from build123d import *
from OCP.BRepFilletAPI import BRepFilletAPI_MakeChamfer

# Parameters (mm, degrees)
BASE_FLANGE1_DEPTH             = 70
SKETCH7_W                      = 25
SKETCH7_H                      = 20
CUT_EXTRUDE1_DEPTH             = 90.017176187
MIRROR10_COPY_1_SKETCH_W       = 25
MIRROR10_COPY_1_SKETCH_H       = 20
MIRROR10_COPY_1_DEPTH          = 90.017176187
FILLET3_R                      = 10
FILLET4_R                      = 2
TAP_DRILL_FOR_4_40_TAP1_D      = 2.2606
SKETCH11_R                     = 5
CUT_EXTRUDE2_DEPTH             = 10
CUT_EXTRUDE3_DEPTH             = 10
CIRPATTERN1_COUNT              = 6
F_5_16_0_3125_DIAMETER_HOLE1_D = 7.9375
TAP_DRILL_FOR_M3X0_5_TAP1_D    = 2.5
CIRPATTERN2_COUNT              = 4
CHAMFER2_SIZE                  = 17
CHAMFER2_SIZE2                 = 9.814954576
FILLET5_R                      = 3
CHAMFER3_SIZE                  = 17
CHAMFER3_SIZE2                 = 9.814954576
FILLET6_R                      = 3


# Sheet-metal steps are written as plain solids
with BuildPart() as part:
    # Sketch2 → Base-Flange1 (new body)
    with BuildSketch(Plane.XY):
        with BuildLine():
            Line((-44.5, 30), (-44.5, 0.7366))
            ThreePointArc((-44.5, 0.7366), (-44.284254855, 0.215745145), (-43.7634, 0))
            Line((-43.7634, 0), (43.7634, 0))
            ThreePointArc((43.7634, 0), (44.284254855, 0.215745145), (44.5, 0.7366))
            Line((44.5, 0.7366), (44.5, 30))
            Line((44.5, 30), (46.0875, 30))
            Line((46.0875, 30), (46.0875, 0.7366))
            ThreePointArc((46.0875, 0.7366), (45.40678687, -0.90678687), (43.7634, -1.5875))
            Line((43.7634, -1.5875), (-43.7634, -1.5875))
            ThreePointArc((-43.7634, -1.5875), (-45.40678687, -0.90678687), (-46.0875, 0.7366))
            Line((-46.0875, 0.7366), (-46.0875, 30))
            Line((-46.0875, 30), (-44.5, 30))
        make_face()
    extrude(amount=BASE_FLANGE1_DEPTH)

    # Sketch7 → Cut-Extrude1 (cut, symmetric)
    with BuildSketch(Plane(origin=(0, 0, 0), x_dir=(1, 0, 0), z_dir=(0, 1, 0))):
        with Locations((-33.5875, -60)):
            Rectangle(SKETCH7_W, SKETCH7_H)
    cut_extrude1 = extrude(amount=CUT_EXTRUDE1_DEPTH, both=True, mode=Mode.SUBTRACT)

    # Mirror9: Cut-Extrude1 across plane
    add(cut_extrude1.mirror(Plane.ZY), mode=Mode.SUBTRACT)

    # Mirror10: Cut-Extrude1 across plane
    add(cut_extrude1.mirror(Plane(origin=(0, 0, 35), x_dir=(1, 0, 0), z_dir=(0, 0, -1))), mode=Mode.SUBTRACT)

    # Mirror10 copy 1 sketch → Mirror10 copy 1 (cut, symmetric)
    with BuildSketch(Plane(origin=(0, 0, 70), x_dir=(-1, 0, 0), z_dir=(0, 1, 0))):
        with Locations((-33.5875, -60)):
            Rectangle(MIRROR10_COPY_1_SKETCH_W, MIRROR10_COPY_1_SKETCH_H)
    extrude(amount=MIRROR10_COPY_1_DEPTH, both=True, mode=Mode.SUBTRACT)

    # Fillet3
    fillet3_edges = [part.edges().sort_by_distance(p)[0] for p in [
        (21.0875, -0.79375, 0),
        (-21.0875, -0.79375, 0),
        (-21.0875, -0.79375, 70),
        (21.0875, -0.79375, 70),
    ]]
    fillet(fillet3_edges, radius=FILLET3_R)

    # Fillet4
    fillet4_edges = [part.edges().sort_by_distance(p)[0] for p in [
        (21.0875, -0.79375, 20),
        (-21.0875, -0.79375, 20),
        (-21.0875, -0.79375, 50),
        (21.0875, -0.79375, 50),
    ]]
    fillet(fillet4_edges, radius=FILLET4_R)

    # Tap Drill for #4-40 Tap1 (through all)
    with Locations(Plane(origin=(0, 0, 0), x_dir=(1, 0, 0), z_dir=(0, 1, 0))):
        with Locations((0.5, -10), (0.5, -60), (-34.5, -35), (35.5, -35), (-14.74, -60), (15.74, -60), (-14.74, -10), (15.74, -10)):
            Hole(TAP_DRILL_FOR_4_40_TAP1_D / 2)

    # Sketch11 → Cut-Extrude2 (cut)
    with BuildSketch(Plane(origin=(0, 0, 0), x_dir=(1, 0, 0), z_dir=(0, 1, 0))):
        with Locations(Location((-0.5, -35, 0), (0, 0, 270))):
            Circle(SKETCH11_R)
    extrude(amount=-CUT_EXTRUDE2_DEPTH, mode=Mode.SUBTRACT)

    # Sketch12 → Cut-Extrude3 (cut)
    with BuildSketch(Plane(origin=(0, 0, 0), x_dir=(1, 0, 0), z_dir=(0, 1, 0))):
        with BuildLine():
            Line((9.5, -33), (19.5, -33))
            ThreePointArc((19.5, -33), (21.5, -35), (19.5, -37))
            Line((19.5, -37), (9.5, -37))
            ThreePointArc((9.5, -37), (7.5, -35), (9.5, -33))
        make_face()
    cut_extrude3 = extrude(amount=-CUT_EXTRUDE3_DEPTH, mode=Mode.SUBTRACT)

    # CirPattern1: Cut-Extrude3 ×6 about axis
    cirpattern1_axis = Axis((-0.5, 0, 35), (0, 1, 0))
    for i in range(1, CIRPATTERN1_COUNT):
        add(cut_extrude3.rotate(cirpattern1_axis, i * 360 / CIRPATTERN1_COUNT), mode=Mode.SUBTRACT)

    # 5/16 (0.3125) Diameter Hole1 (through all)
    with Locations(Plane(origin=(46.0875, 0, 0), x_dir=(0, 0, -1), z_dir=(1, 0, 0))):
        with Locations((-35, 20)):
            Hole(F_5_16_0_3125_DIAMETER_HOLE1_D / 2)

    # Tap Drill for M3x0.5 Tap1 (through all)
    with Locations(Plane(origin=(46.0875, 0, 0), x_dir=(0, 0, -1), z_dir=(1, 0, 0))):
        with Locations((-35, 13)):
            tap_drill_for_m3x0_5_tap1 = Hole(TAP_DRILL_FOR_M3X0_5_TAP1_D / 2)

    # CirPattern2: Tap Drill for M3x0.5 Tap1 ×4 about axis
    cirpattern2_axis = Axis((0, 20, 35), (1, 0, 0))
    for i in range(1, CIRPATTERN2_COUNT):
        add(tap_drill_for_m3x0_5_tap1.rotate(cirpattern2_axis, i * 360 / CIRPATTERN2_COUNT), mode=Mode.SUBTRACT)

    # Chamfer2: one chamfer whose edges measure the first distance from different faces: ONE call of the kernel's chamfer builder (chamfer() names one face for all edges)
    chamfer2_edges_1 = [part.edges().sort_by_distance(p)[0] for p in [
        (45.29375, 30, 20),
    ]]
    chamfer2_side_1 = [part.faces().sort_by_distance(p)[0] for p in [
        (33.42545, -0.390739063, 20),
    ]]
    chamfer2_edges_2 = [part.edges().sort_by_distance(p)[0] for p in [
        (45.29375, 30, 50),
    ]]
    chamfer2_side_2 = [part.faces().sort_by_distance(p)[0] for p in [
        (33.42545, -0.390739063, 50),
    ]]
    chamfer2 = BRepFilletAPI_MakeChamfer(part.part.solid().wrapped)
    for e in chamfer2_edges_1:
        chamfer2.Add(CHAMFER2_SIZE, CHAMFER2_SIZE2, e.wrapped, chamfer2_side_1[0].wrapped)  # the first distance lies on this face
    for e in chamfer2_edges_2:
        chamfer2.Add(CHAMFER2_SIZE, CHAMFER2_SIZE2, e.wrapped, chamfer2_side_2[0].wrapped)  # the first distance lies on this face
    add(Compound.cast(chamfer2.Shape()), mode=Mode.REPLACE)

    # Fillet5
    fillet5_edges = [part.edges().sort_by_distance(p)[0] for p in [
        (45.29375, 13, 20),
        (45.29375, 30, 40.185045424),
        (45.29375, 30, 29.814954576),
        (45.29375, 13, 50),
    ]]
    fillet(fillet5_edges, radius=FILLET5_R)

    # Chamfer3: one chamfer whose edges measure the first distance from different faces: ONE call of the kernel's chamfer builder (chamfer() names one face for all edges)
    chamfer3_edges_1 = [part.edges().sort_by_distance(p)[0] for p in [
        (-45.29375, 30, 20),
    ]]
    chamfer3_side_1 = [part.faces().sort_by_distance(p)[0] for p in [
        (-33.42545, -0.390739063, 20),
    ]]
    chamfer3_edges_2 = [part.edges().sort_by_distance(p)[0] for p in [
        (-45.29375, 30, 50),
    ]]
    chamfer3_side_2 = [part.faces().sort_by_distance(p)[0] for p in [
        (-33.42545, -0.390739063, 50),
    ]]
    chamfer3 = BRepFilletAPI_MakeChamfer(part.part.solid().wrapped)
    for e in chamfer3_edges_1:
        chamfer3.Add(CHAMFER3_SIZE, CHAMFER3_SIZE2, e.wrapped, chamfer3_side_1[0].wrapped)  # the first distance lies on this face
    for e in chamfer3_edges_2:
        chamfer3.Add(CHAMFER3_SIZE, CHAMFER3_SIZE2, e.wrapped, chamfer3_side_2[0].wrapped)  # the first distance lies on this face
    add(Compound.cast(chamfer3.Shape()), mode=Mode.REPLACE)

    # Fillet6
    fillet6_edges = [part.edges().sort_by_distance(p)[0] for p in [
        (-45.29375, 13, 50),
        (-45.29375, 30, 29.814954576),
        (-45.29375, 30, 40.185045424),
        (-45.29375, 13, 20),
    ]]
    fillet(fillet6_edges, radius=FILLET6_R)


solid = part.part
Read the model definition and answer for the solid it produces. Units are mm, in the model's axes. A direction names the side the tool comes from. Give positions to 0.01 mm unless a question says otherwise; leave off trailing zeros. Loops run counter-clockwise (first coordinate to the right, second up) from the corner with the lowest first, then second, coordinate; pieces in that order, holes last. Notation, with made-up numbers: (72, -12.5) -> (125, -12.5) arc R13 cw to (125, -8.5) -> close; hole circle Ø4 at (86.25, 10.5). An arc over 180 degrees is marked (long way). Use a Markdown table: item, result.
Q1. Determine the mould class of faces 1 (the face through (-8.5, -0.8, 35)), 2 (the face through (46.088, 15.6, 34.8)), 3 (the face through (-38.9, -0.3, 20)) for opening direction X: pulls with the +X half, pulls with the -X half, needs draft (parallel to the pull), parting line crosses it, or undercut.
Solved:
| item | result |
|---|---|
| face 1 | undercut |
| face 2 | pulls with the +X half |
| face 3 | needs draft |
Q2. A tool of negligible diameter and unlimited length cuts with its end or side. For faces 4 (the face through (45.28, 14.24, 34.84)), 5 (the face through (-9.697, -0.783, 23.07)), 6 (the face through (-44.5, 15.6, 34.8)), from which of +Z, -Z, +X, -X, +Y, -Y can it reach the whole face along a straight path? Write none if from no direction.
Solved:
| item | result |
|---|---|
| face 4 | +X, -X |
| face 5 | +Y, -Y |
| face 6 | +Z, -Z, +Y |
Q3. Section B-B, the plane x = 15.74 is taken. Determine the outline of the cut face in (y, z).
Solved:
| item | result |
|---|---|
| outline | (-1.59, 1.15) -> (0, 1.15) -> (0, 8.87) -> (-1.59, 8.87) -> close; (-1.59, 11.13) -> (0, 11.13) -> (0, 33) -> (-1.59, 33) -> close; (-1.59, 37) -> (0, 37) -> (0, 58.87) -> (-1.59, 58.87) -> close; (-1.59, 61.13) -> (0, 61.13) -> (0, 68.85) -> (-1.59, 68.85) -> close |
Q4. Each of these flat-tipped pins is pushed along its axis until it touches: pin 1 (2 mm diameter, centred on x = -34.5, z = 35, fed in from -Y); pin 2 (2.5 mm diameter, centred on x = 0.5, z = 60, fed in from +Y); pin 3 (4 mm diameter, centred on y = 27, z = 35, fed in from +X); pin 4 (1.7 mm diameter, centred on y = -0.5, z = 55, fed in from -X). Where does it stop, or does it pass through?
Solved:
| item | result |
|---|---|
| pin 1 | passes through |
| pin 2 | stops at y = 0 |
| pin 3 | stops at x = 46.09 |
| pin 4 | stops at x = -21.09 |
Q5. Section A-A, the plane x = 35.5 is taken. Determine the outline of the cut face in (y, z).
Solved:
| item | result |
|---|---|
| outline | (-1.59, 20) -> (0, 20) -> (0, 33.87) -> (-1.59, 33.87) -> close; (-1.59, 36.13) -> (0, 36.13) -> (0, 50) -> (-1.59, 50) -> close |
Q6. Section C-C, the plane y = 20 is taken. Count the separate pieces of the cut face and the enclosed holes in it, then the cut area to 3 significant figures.
Solved:
| item | result |
|---|---|
| separate pieces | 8 |
| enclosed holes | 0 |
| area | 28.5 mm^2 |
Q7. Section D-D, the plane z = 24 is taken. Determine the outline of the cut face in (x, y), then the cut area to 3 significant figures.
Solved:
| item | result |
|---|---|
| outline | (-46.09, 0.74) arc R2.32 ccw to (-43.76, -1.59) -> (-9.16, -1.59) -> (-9.16, 0) -> (-43.76, 0) arc R0.74 cw to (-44.5, 0.74) -> (-44.5, 19.93) -> (-46.09, 19.93) -> close; (-4.54, -1.59) -> (3.54, -1.59) -> (3.54, 0) -> (-4.54, 0) -> close; (8.16, -1.59) -> (43.76, -1.59) arc R2.32 ccw to (46.09, 0.74) -> (46.09, 19.93) -> (44.5, 19.93) -> (44.5, 0.74) arc R0.74 cw to (43.76, 0) -> (8.16, 0) -> close |
| area | 193 mm^2 |
Q8. Find the intervals of material crossed by line 1 along Z through (x, y) = (15.74, -0.55); line 2 along X through (y, z) = (12, 40); line 3 along Z through (x, y) = (-14.74, -0.6), in increasing order.
Solved:
| item | result |
|---|---|
| line 1 | z = 1.15 to 8.87, 11.13 to 33, 37 to 58.87, 61.13 to 68.85 |
| line 2 | x = -46.09 to -44.5, 44.5 to 46.09 |
| line 3 | z = 0.69 to 8.87, 11.13 to 33, 37 to 58.87, 61.13 to 69.31 |
